Autodesk Inventor part; units mm, degrees
ref_plane "YZ Plane" through (0, 0, 0) normal (1, 0, 0) x (0, 1, 0)
ref_plane "XZ Plane" through (0, 0, 0) normal (0, 1, 0) x (-1, 0, 0)
ref_plane "XY Plane" through (0, 0, 0) normal (0, 0, 1) x (1, 0, 0)
sketch "Sketch1" plane through (0, 0, 0) normal (0, 0, 1) x (1, 0, 0)
  line L0 (-24.5, 24.5) -> (24.5, 24.5)
  line L1 (24.5, 24.5) -> (24.5, -24.5)
  line L2 (24.5, -24.5) -> (-24.5, -24.5)
  line L3 (-24.5, -24.5) -> (-24.5, 24.5)
  point P0 (0, 0)
  point P1 (-24.5, 0)
  point P2 (0, 24.5)
  dimension "Width" = 49
  dimension "Height" = 49
extrude "Extrusion1" add sketch "Sketch1" along normal blind 20
sketch "Sketch2" plane through (0, 0, 20) normal (0, 0, 1) x (1, 0, 0)
  line L0 (24.5, 24.5) -> (24.5, -24.5)
  line L1 (-24.5, 24.5) -> (24.5, 24.5)
  line L2 (-24.5, -24.5) -> (-24.5, 24.5)
  line L3 (24.5, -24.5) -> (-24.5, -24.5)
  line L4 (19.5, 19.5) -> (19.5, -19.5)
  line L5 (19.5, -19.5) -> (-19.5, -19.5)
  line L6 (-19.5, -19.5) -> (-19.5, 19.5)
  line L7 (-19.5, 19.5) -> (19.5, 19.5)
  point P0 (0, 0)
  dimension "d4" = 5
  dimension "d5" = 39
  dimension "d6" = 39
hole "Hole1" at (-19.5, -19.5, 20) direction (0, 0, -1) diameter 6 end through all
pattern_linear "Rectangular Pattern1" count 2 spacing 39 along (1, 0, 0) count 2 spacing 39 along (0, 1, 0) of "Hole1"
sketch "Sketch3" plane through (0, 0, 0) normal (1, 0, 0) x (0, 1, 0)
  line L0 (-24.5, 20) -> (24.5, 20)
  line L1 (0, 20) -> (0, 28)
  line L2 (0, 28) -> (20.5, 28)
  line L3 (20.5, 28) -> (20.5, 26)
  line L4 (20.5, 26) -> (17.5, 26)
  line L5 (17.5, 26) -> (17.5, 22)
  line L6 (17.5, 22) -> (20.5, 22)
  line L7 (20.5, 22) -> (20.5, 20)
  point P0 (0, 0)
  dimension "d25" = 8
  dimension "d26" = 20.5
  dimension "d27" = 2
  dimension "d28" = 4
  dimension "d29" = 17.5
revolve "Revolution1" add sketch "Sketch3" angle 360 about axis through (0, 0, 20) along (0, 0, 1)
sketch "Sketch4" plane through (-24.5, 24.5, 0) normal (0, 1, 0) x (1, 0, 0)
  line L0 (0, -20) -> (49, -20)
  line L1 (0, 0) -> (0, -20)
  line L2 (24.5, -20) -> (24.5, -10)
  point P0 (24.5, 0)
  dimension "d31" = 10
hole "Hole4" at (0, 24.5, 10) direction (0, -1, 0) diameter 4.134 depth 14 tip angle 118
ref_plane "Work Plane3" through (0, 24.5, 10) normal (0, 0, 1) x (0, -1, 0)
sketch "Sketch7" plane through (0, 0, 28) normal (0, 0, 1) x (1, 0, 0)
  circle A0 centre (0, 0) radius 20.5
  line L0 (0, 0) -> (0, 12.5)
  dimension "d56" = 12.5
hole "Hole5" at (0, 12.5, 28) direction (0, 0, -1) diameter 4 depth 18
hole "Hole6" at (0, 0, 28) direction (0, 0, -1) diameter 14 end through all
equation "\"Height\" = Width"
equation "\"d16\" = d5"
equation "\"d19\" = d6"
properties part number "TU-002" material "Steel, Mild"
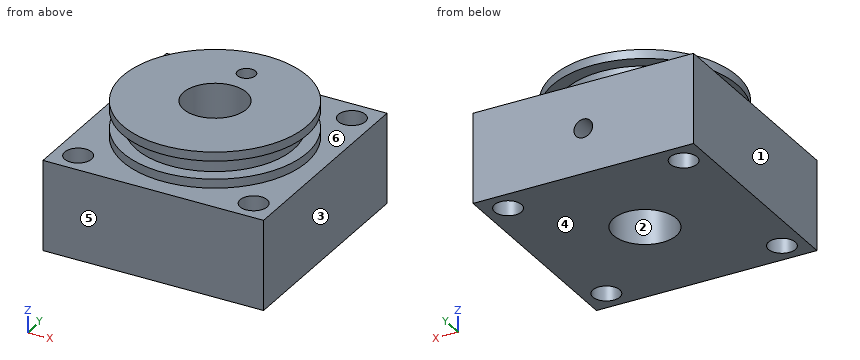
Build history of the part. All positions in model axes, mm. Face numbers are marked on the shaded views. A direction names the side the tool comes from. Coordinates: 2 decimals unless noted, no trailing zeros. Write each loop counter-clockwise with the first axis right and the second up, starting at its lowest first coordinate (ties: lowest second). Pieces come first, ordered by that corner, then holes.
(1) Cut at B-B on z = 6.25. List the corners of the cut face in (x, y), and give its area (3 significant figures).
(2) Cut at D-D on z = 16. List the corners of the cut face in (x, y), and give its area (3 significant figures).
(3) Pin check, flat tips, straight feed: pin 1 Ø6.5 at (x, y) = (0, 12.5) entering from +Z; pin 2 Ø8 at (x, y) = (-19.5, -19.5) entering from +Z; pin 3 Ø12.5 at (x, y) = (0, 0) entering from +Z. Stop position of each tip, or through.
(4) Cut at A-A on y = 0. List the corners of the cut face in (x, z).
(5) Cut at C-C on x = 0. List the corners of the cut face in (y, z).
(6) Mould opens along X. For the marked faces 1, 2, 3 and 4 say: pulls with the +X half, pulls with the -X half, needs draft (parallel to the pull), parting line crosses it, or undercut.
(7) Drill centre lines: line 1 (Y direction, x = 0, z = 16); line 2 (Y direction, x = 0, z = 20.5); line 3 (X direction, y = 19.5, z = 7). Where is each one in solid material? Low to high.
(8) 3-axis set-ups, long thin cutter, end or side, ignore diameter. For the marked faces 5 and 6: which of +Z, -Z, +X, -X, +Y, -Y reach the whole face in a straight line?
Working result:
1. outline: (-24.5, -24.5) - (24.5, -24.5) - (24.5, 24.5) - (-24.5, 24.5) - close; hole circle Ø6 at (-19.5, -19.5); hole circle Ø6 at (-19.5, 19.5); hole circle Ø14 at (0, 0); hole circle Ø6 at (19.5, -19.5); hole circle Ø6 at (19.5, 19.5)
1. area: 2,130 mm2
2. outline: (-24.5, -24.5) - (24.5, -24.5) - (24.5, 24.5) - (-24.5, 24.5) - close; hole circle Ø6 at (-19.5, -19.5); hole circle Ø6 at (-19.5, 19.5); hole circle Ø14 at (0, 0); hole circle Ø4 at (0, 12.5); hole circle Ø6 at (19.5, -19.5); hole circle Ø6 at (19.5, 19.5)
2. area: 2,120 mm2
3. pin 1: stops at z = 28
3. pin 2: stops at z = 20
3. pin 3: passes through
4. outline: (-24.5, 0) - (-7, 0) - (-7, 28) - (-20.5, 28) - (-20.5, 26) - (-17.5, 26) - (-17.5, 22) - (-20.5, 22) - (-20.5, 20) - (-24.5, 20) - close; (7, 0) - (24.5, 0) - (24.5, 20) - (20.5, 20) - (20.5, 22) - (17.5, 22) - (17.5, 26) - (20.5, 26) - (20.5, 28) - (7, 28) - close
5. outline: (-24.5, 0) - (-7, 0) - (-7, 28) - (-20.5, 28) - (-20.5, 26) - (-17.5, 26) - (-17.5, 22) - (-20.5, 22) - (-20.5, 20) - (-24.5, 20) - close; (7, 0) - (24.5, 0) - (24.5, 7.93) - (10.5, 7.93) - (9.26, 10) - (10.5, 12.07) - (10.5, 28) - (7, 28) - close; (14.5, 12.07) - (24.5, 12.07) - (24.5, 20) - (20.5, 20) - (20.5, 22) - (17.5, 22) - (17.5, 26) - (20.5, 26) - (20.5, 28) - (14.5, 28) - close
6. face 1: pulls with the -X half
6. face 2: undercut
6. face 3: pulls with the +X half
6. face 4: needs draft
7. line 1: y = -24.5 to -7, 7 to 10.5, 14.5 to 24.5
7. line 2: y = -20.5 to -7, 7 to 10.5, 14.5 to 20.5
7. line 3: x = -24.5 to -22.5, -16.5 to 16.5, 22.5 to 24.5
8. face 5: +Z, -Z, +X, -X, -Y
8. face 6: +Z
